```python
from build123d import *

# Parameters (mm, degrees)
F0_W     = 19.05
F0_H     = 19.05
F1_DEPTH = 6.35
F2_W     = 19.05
F2_H     = 25.4
F3_DEPTH = 6.35
F4_R     = 5.08
F5_R     = 5.08
F6_SIZE  = 5.08
F7_R     = 4.42696
F8_DEPTH = 6.351


with BuildPart() as f1:
    # F0 (on Front) → F1 (new body)
    with BuildSketch(Plane.XZ):
        with Locations((-23.501792, 18.51008)):
            Rectangle(F0_W, F0_H)
    extrude(amount=F1_DEPTH)

    # F2 (on face) → F3 (join)
    with BuildSketch(Plane(origin=(0, 0, 8.98508), x_dir=(1, 0, 0), z_dir=(0, 0, -1))):
        with Locations((-23.501792, 12.7)):
            Rectangle(F2_W, F2_H)
    extrude(amount=F3_DEPTH)

    # F4
    f4_edges = [f1.edges().sort_by_distance(p)[0] for p in [
        (-13.976792, -25.4, 5.81008),
    ]]
    fillet(f4_edges, radius=F4_R)

    # F5
    f5_edges = [f1.edges().sort_by_distance(p)[0] for p in [
        (-33.026792, -25.4, 5.81008),
    ]]
    fillet(f5_edges, radius=F5_R)

    # F6
    f6_edges = [f1.edges().sort_by_distance(p)[0] for p in [
        (-13.976792, -3.175, 28.03508),
        (-33.026792, -3.175, 28.03508),
    ]]
    chamfer(f6_edges, length=F6_SIZE)

    # F7 (on face) → F8 (cut, through all)
    with BuildSketch(Plane.XY.offset(8.98508)):
        with Locations((-22.985389, -15.249236)):
            Circle(F7_R)
    extrude(amount=-F8_DEPTH, mode=Mode.SUBTRACT)


solid = f1.part
```
Geometry check sheet. Reference: the model listing, model coordinates, mm. A direction names the side the tool comes from. Coordinates: 2 decimals unless noted, no trailing zeros. Write each loop counter-clockwise with the first axis right and the second up, starting at its lowest first coordinate (ties: lowest second). Pieces come first, ordered by that corner, then holes. Notation, with made-up numbers: (61, 63.25) -> (120, 63.25) arc R14 ccw to (120, 76.25) -> close; hole circle Ø2 at (25.25, 38.25). An arc over 180 degrees is marked (long way). Use CSV: the item, a comma, the result in double quotes. Start each with the question number.
Item 1: Cross-section at C-C, the plane y = -2.5. Record the cut outline in (x, z).
Item 2: Cross-section at D-D, the plane z = 20.25. Record the cut outline in (x, y).
Item 3: Depth check by flat-ended pin: pin 1 Ø4 at (x, z) = (-30.5, 5.5) entering from +Y; pin 2 Ø1.5 at (y, z) = (-5.5, 25) entering from -X; pin 3 Ø5 at (x, z) = (-31, 20) entering from -Y. Enter the tip coordinate at first touch or a pass-through.
Item 4: Mould release check, pull along X, two halves, no side actions. Record for faces 3 (the cylindrical face through (-23.95, -19.57, 5.85)), 4 (the flat face through (-13.977, -6, 11)), 5 (the flat face through (-24, -25.4, 6)): released by +X, released by -X, zero draft, split by the parting line, or undercut.
Item 5: Set-up check for faces 1 (the flat face through (-24, 0, 16)), 2 (the flat face through (-24, -6.35, 19)): record each of +Z, -Z, +X, -X, +Y, -Y from which the full face is reachable in a straight line by a thin tool's end or side.
Item 6: Thickness scan on line 1 (Y direction, x = -18.25, z = 24.5); line 2 (Z direction, x = -22.5, y = -9.5); line 3 (Y direction, x = -24.5, z = 6). Record the ranges inside material, lowest first.
Item 7: Cross-section at A-A, the plane y = -12.25. Record the cut outline in (x, z), plus the area to 3 significant figures.
Item 8: Cross-section at B-B, the plane x = -21.5. Record the cut outline in (y, z).
Answers:
1,outline,"(-33.03, 2.64) -> (-13.98, 2.64) -> (-13.98, 22.96) -> (-19.06, 28.04) -> (-27.95, 28.04) -> (-33.03, 22.96) -> close"
2,outline,"(-33.03, -6.35) -> (-13.98, -6.35) -> (-13.98, 0) -> (-33.03, 0) -> close"
3,pin 1,"y = 0"
3,pin 2,"x = -31.73"
3,pin 3,"y = -6.35"
4,face 3,"undercut"
4,face 4,"released by +X"
4,face 5,"zero draft"
5,face 1,"+Z, -Z, +X, -X, +Y"
5,face 2,"+Z, +X, -X, -Y"
6,line 1,"-6.35 to 0"
6,line 2,"2.64 to 8.99"
6,line 3,"-25.4 to -19.41, -11.09 to 0"
7,outline,"(-33.03, 2.64) -> (-26.24, 2.64) -> (-26.24, 8.99) -> (-33.03, 8.99) -> close; (-19.73, 2.64) -> (-13.98, 2.64) -> (-13.98, 8.99) -> (-19.73, 8.99) -> close"
7,area,"79.6 mm^2"
8,outline,"(-25.4, 2.64) -> (-19.42, 2.64) -> (-19.42, 8.99) -> (-25.4, 8.99) -> close; (-11.08, 2.64) -> (0, 2.64) -> (0, 28.04) -> (-6.35, 28.04) -> (-6.35, 8.99) -> (-11.08, 8.99) -> close"
